For this review, use the dimensioned drawing (mm, ordinates from the lowest corner) and the shaded views. A direction names the side the tool comes from. Coordinates: 2 decimals unless noted, no trailing zeros. Write each loop counter-clockwise with the first axis right and the second up, starting at its lowest first coordinate (ties: lowest second). Pieces come first, ordered by that corner, then holes. Notation, with made-up numbers: (26.25, 51) - (78.25, 51) arc R30 ccw to (78.25, 83) - close; hole circle Ø2 at (76, 44). An arc over 180 degrees is marked (long way). Use one line per item in the form item = value. Start each with the question number.
1) Mouldability with a two-part tool opening along X and no side actions: class the marked faces 1, 2 and 3 as pulls with the +X half, pulls with the -X half, needs draft (parallel to the pull), parting line crosses it, or undercut.
2) We need section C-C (y = 32). Give the boundary of the cut face in (x, z).
3) For L1, parallel to Y at x = 7.5, z = 13.15; L2, parallel to X at y = 19.5, z = 13; L3, parallel to X at y = 30.5, z = 17, list the stretches that pass through material, from the lowest coordinate up. Write a range as from..to.
4) We need section A-A (x = 30.5). Give the boundary of the cut face in (y, z).
5) We need section B-B (x = 19). Give the boundary of the cut face in (y, z).
6) Insertion check: P1, Ø5, axis at x = 11, z = 5, coming from the +Y side; P2, Ø2.5, axis at x = 30.5, y = 24.3, coming from the +Z side; P3, Ø4, axis at x = 34, y = 17, coming from the -Z side. Each pin has a flat end and moves straight along its axis. Give the tip position at first contact, or say it passes through.
7) Tool access review of the marked faces 4, 5, 6, 7 and 8: name each direction out of +Z, -Z, +X, -X, +Y, -Y from which nothing blocks a thin tool from reaching the whole face with its end or side.
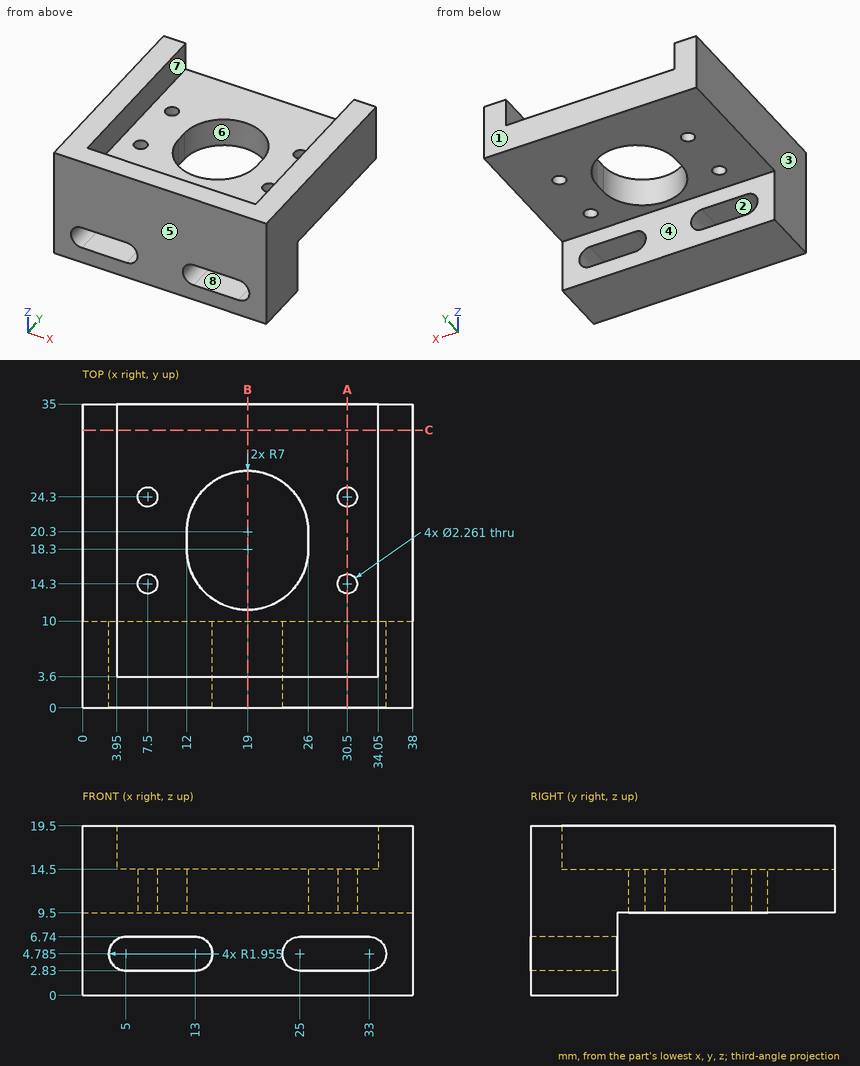
Determined:
q1.face_1 = needs draft
q1.face_2 = undercut
q1.face_3 = pulls with the -X half
q2.outline = (0, 9.5) - (38, 9.5) - (38, 19.5) - (34.05, 19.5) - (34.05, 14.5) - (3.95, 14.5) - (3.95, 19.5) - (0, 19.5) - close
q3.L1 = 0..13.17, 15.43..23.17, 25.43..35
q3.L2 = 0..12, 26..38
q3.L3 = 0..3.95, 34.05..38
q4.outline = (0, 0) - (10, 0) - (10, 2.83) - (0, 2.83) - close; (0, 6.74) - (10, 6.74) - (10, 9.5) - (13.17, 9.5) - (13.17, 14.5) - (3.6, 14.5) - (3.6, 19.5) - (0, 19.5) - close; (15.43, 9.5) - (23.17, 9.5) - (23.17, 14.5) - (15.43, 14.5) - close; (25.43, 9.5) - (35, 9.5) - (35, 14.5) - (25.43, 14.5) - close
q5.outline = (0, 0) - (10, 0) - (10, 9.5) - (11.3, 9.5) - (11.3, 14.5) - (3.6, 14.5) - (3.6, 19.5) - (0, 19.5) - close; (27.3, 9.5) - (35, 9.5) - (35, 14.5) - (27.3, 14.5) - close
q6.P1 = 10
q6.P2 = 14.5
q6.P3 = 9.5
q7.face_4 = -Z, +X, -X, +Y
q7.face_5 = +Z, -Z, +X, -X, -Y
q7.face_6 = +Z, -Z
q7.face_7 = +Z, +Y
q7.face_8 = +Y, -Y
